```python
from build123d import *

# Parameters (mm, degrees)
F0_R      = 80.4673318477
F1_DEPTH  = 48.26
F4_DEPTH  = 25.4
F6_DEPTH  = 25.4
F8_DEPTH  = 48.26
F9_DEPTH  = 2.54
F11_DEPTH = 482.6
F12_R     = 38.1
F13_DEPTH = 127


with BuildPart() as f1:
    # F0 (on Top) → F1 (new body)
    with BuildSketch(Plane.XY):
        with BuildLine():
            Line((1010.2228706353, 495.3), (1010.2228706353, 0))
            Line((1010.2228706353, 0), (2343.7228706353, 0))
            ThreePointArc((2343.7228706353, 0), (2424.5451757249, 33.4776949104), (2458.0228706353, 114.3))
            Line((2458.0228706353, 114.3), (2458.0228706353, 381))
            ThreePointArc((2458.0228706353, 381), (2424.5451757249, 461.8223050896), (2343.7228706353, 495.3))
            Line((2343.7228706353, 495.3), (1010.2228706353, 495.3))
        make_face()
        with Locations((1645.2228706353, 291.9926941395)):
            Circle(F0_R, mode=Mode.SUBTRACT)
        with BuildLine():
            ThreePointArc((1962.7228706353, 244.6997875276), (1899.2228706353, 308.1997875276), (1962.7228706353, 371.6997875276))
            Line((1962.7228706353, 371.6997875276), (2343.7228706353, 371.6997875276))
            ThreePointArc((2343.7228706353, 371.6997875276), (2407.2228706353, 308.1997875276), (2343.7228706353, 244.6997875276))
            Line((2343.7228706353, 244.6997875276), (1962.7228706353, 244.6997875276))
        make_face(mode=Mode.SUBTRACT)
    extrude(amount=F1_DEPTH)

    # F3 (on face) → F4 (join)
    with BuildSketch(Plane.XZ):
        Polygon((1008.9916278534, 193.5739982539), (1017.166601884, 158.4598601468), (1576.1663705805, 481.1985270807), (1558.9177592565, 511.0739982539), align=None)
        with BuildLine():
            ThreePointArc((1017.166601884, 50.3464564681), (985.9569505255, 104.4031583075), (1017.166601884, 158.4598601468))
            Line((1017.166601884, 158.4598601468), (1008.9916278534, 193.5739982539))
            ThreePointArc((1008.9916278534, 193.5739982539), (953.1116278534, 96.7869991269), (1008.9916278534, 0))
            Line((1008.9916278534, 0), (1017.166601884, 50.3464564681))
        make_face()
    extrude(amount=-F4_DEPTH)



with BuildPart() as f6:
    # F5 (on face) → F6 (new body)
    with BuildSketch(Plane(origin=(0, 495.3, 0), x_dir=(-1, 0, 0), z_dir=(0, 1, 0))):
        with BuildLine():
            Line((-962.622620171, 212.8763377291), (-986.752620171, 171.0819517425))
            ThreePointArc((-986.752620171, 171.0819517425), (-947.7007055922, 99.9659962012), (-1010.2228706353, 48.26))
            Line((-1010.2228706353, 48.26), (-1010.2228706353, 0))
            ThreePointArc((-1010.2228706353, 0), (-901.1562407602, 87.3721372872), (-962.622620171, 212.8763377291))
        make_face()
        Polygon((-1512.5487515741, 530.3763377291), (-1536.6787515741, 488.5819517425), (-986.752620171, 171.0819517425), (-962.622620171, 212.8763377291), align=None)
    extrude(amount=-F6_DEPTH)


with BuildPart() as f1_1:
    add(f1.part)

    add(f6.part)  # F8 merges F6
    # F7 (on face) → F8 (join)
    with BuildSketch(Plane(origin=(148.4774968738, 0, -257.170568366), x_dir=(0.8660254038, 0, 0.5), z_dir=(-0.5, 0, 0.8660254038))):
        with BuildLine():
            Line((1569.96836326, 495.3), (940.0938121902, 495.3))
            Line((940.0938121902, 495.3), (940.0938121902, 0))
            Line((940.0938121902, 0), (1569.96836326, 0))
            ThreePointArc((1569.96836326, 0), (1659.7709244707, 37.1974387893), (1696.96836326, 127))
            Line((1696.96836326, 127), (1696.96836326, 368.3))
            ThreePointArc((1696.96836326, 368.3), (1659.7709244707, 458.1025612107), (1569.96836326, 495.3))
        make_face()
    extrude(amount=-F8_DEPTH)

    # F7 (on face) → F9 (join)
    with BuildSketch(Plane(origin=(148.4774968738, 0, -257.170568366), x_dir=(0.8660254038, 0, 0.5), z_dir=(-0.5, 0, 0.8660254038))):
        with BuildLine():
            Line((1569.96836326, 495.3), (940.0938121902, 495.3))
            Line((940.0938121902, 495.3), (940.0938121902, 0))
            Line((940.0938121902, 0), (1569.96836326, 0))
            ThreePointArc((1569.96836326, 0), (1659.7709244707, 37.1974387893), (1696.96836326, 127))
            Line((1696.96836326, 127), (1696.96836326, 368.3))
            ThreePointArc((1696.96836326, 368.3), (1659.7709244707, 458.1025612107), (1569.96836326, 495.3))
        make_face()
    extrude(amount=F9_DEPTH)

    # F10 (on face) → F11 (join)
    with BuildSketch(Plane.XZ.offset(-469.9)):
        with BuildLine():
            Line((986.752620171, 171.0819517425), (962.622620171, 212.8763377291))
            ThreePointArc((962.622620171, 212.8763377291), (901.1562407602, 87.3721372872), (1010.2228706353, 0))
            Line((1010.2228706353, 0), (1010.2228706353, 48.26))
            ThreePointArc((1010.2228706353, 48.26), (947.7007055922, 99.9659962012), (986.752620171, 171.0819517425))
        make_face()
    extrude(amount=F11_DEPTH)

    # F12 (on face) → F13 (cut, symmetric)
    with BuildSketch(Plane(origin=(147.2074968738, 0, -254.9708638404), x_dir=(0.8660254038, 0, 0.5), z_dir=(-0.5, 0, 0.8660254038))):
        with Locations((1468.36836326, 342.9)):
            Circle(F12_R)
        with Locations((1468.36836326, 192.6162540913)):
            Circle(F12_R)
    extrude(amount=F13_DEPTH, both=True, mode=Mode.SUBTRACT)


solid = f1_1.part
```
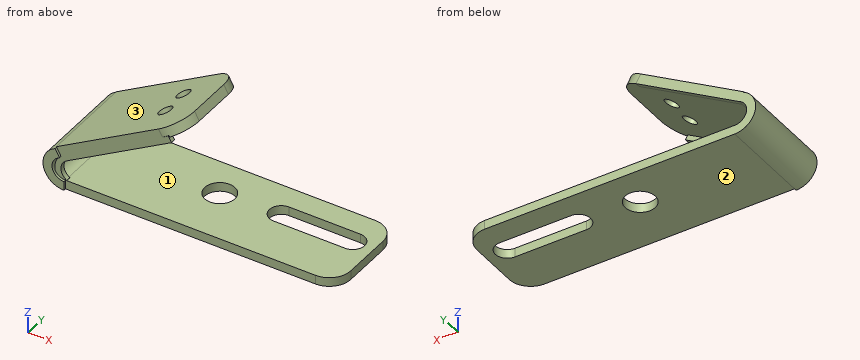
Work out the finished part from the listing and answer in its coordinate system (mm). Face numbers are marked on the shaded views. Coordinates: 2 decimals unless noted, no trailing zeros. Order: outer loops, then holes, each group sorted by start corner. A loop starts at its lowest first (then second) coordinate and runs counter-clockwise, first axis right, second up. Notation, with made-up numbers: M -16,67 L 28,67 A16 ccw 28,96 Z; hole C 74.25,-5.5 d7. An arc over 180 degrees is marked long. Use CSV: the item, a comma, the result in double quotes.
1) Determine the mould class of the marked faces 1, 2 and 3 for opening direction Z: released by +Z, released by -Z, zero draft, split by the parting line, or undercut.
Worked out:
face 1,"undercut"
face 2,"released by -Z"
face 3,"released by +Z"
2) Section C-C on y = 89 is taken. Write down the section's boundary in (x, z), plus the area to 3 significant figures.
Worked out:
outline,"M 961.35,215.08 L 962.62,212.88 A111.76 ccw 1010.22,0 L 2455.19,0 L 2455.19,48.26 L 1010.22,48.26 A63.65 cw 986.75,171.08 L 1637.19,546.61 L 1611.79,590.6 Z"
area,"119,000 mm^2"
3) Consider line 1 (Z direction, x = 2041, y = 463); line 2 (Z direction, x = 1279, y = 172.5); line 3 (Z direction, x = 1108, y = 73). Determine where each line is inside the solid, lowest interval first. Write a range as [from, to].
Worked out:
line 1,"z = [0, 48.26]"
line 2,"z = [0, 48.26], [339.81, 398.47]"
line 3,"z = [0, 48.26], [241.08, 299.74]"
4) Section B-B on z = 109.5 is taken. Write down the section's boundary in (x, y).
Worked out:
outline,"M 898.49,-12.7 L 946.62,-12.7 L 946.62,495.3 L 898.49,495.3 Z; M 953.84,0 L 986.17,0 L 986.17,25.4 L 953.84,25.4 Z"
5) Flat-ended cylindrical pins translate along their axes: pin 1 Ø4 at (y, z) = (-4, 25.5) entering from +X; pin 2 Ø8 at (y, z) = (332.5, 278.5) entering from +X; pin 3 Ø14.5 at (x, z) = (2201.5, 15.5) entering from -Y. Find the tip coordinate at first contact, or state that the pin passes through.
Worked out:
pin 1,"stops at x = 1010.22"
pin 2,"stops at x = 1179.73"
pin 3,"stops at y = 0"
6) Section A-A on x = 2161.5 is taken. Write down the section's boundary in (y, z), plus the area to 3 significant figures.
Worked out:
outline,"M 0,0 L 244.7,0 L 244.7,48.26 L 0,48.26 Z; M 371.7,0 L 495.3,0 L 495.3,48.26 L 371.7,48.26 Z"
area,"17,800 mm^2"
7) Section D-D on z = 342.5 is taken. Write down the section's boundary in (x, y), plus the area to 3 significant figures.
Worked out:
outline,"M 1182.06,0 L 1335.93,0 L 1335.93,25.4 L 1283.66,25.4 L 1283.66,495.3 L 1182.06,495.3 Z"
area,"51,700 mm^2"
